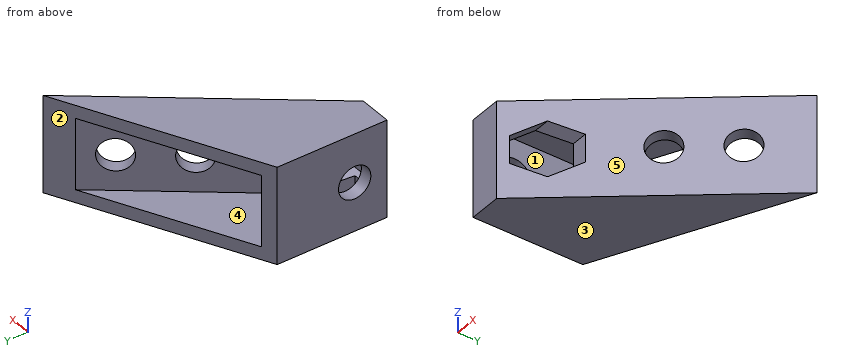
Autodesk Inventor part; units mm, degrees
ref_plane "YZ Plane" through (0, 0, 0) normal (1, 0, 0) x (0, 1, 0)
ref_plane "XZ Plane" through (0, 0, 0) normal (0, 1, 0) x (-1, 0, 0)
ref_plane "XY Plane" through (0, 0, 0) normal (0, 0, 1) x (1, 0, 0)
sketch "Skizze1" plane through (0, 0, 0) normal (0, 0, 1) x (1, 0, 0)
  line L0 (0, 0) -> (0, 17)
  line L1 (0, 0) -> (40, 0) construction
  line L2 (0, 0) -> (5, 0)
  line L3 (5, 0) -> (29.6265, 31.5204)
  line L4 (29.6265, 31.5204) -> (0, 17)
  dimension "d0" = 17
  dimension "d46" = 5
  dimension "d48" = 40
extrude "Extrusion1" add sketch "Skizze1" along normal blind 15
hole "Bohrung1" at (0, 5, 7.5) direction (1, 0, 0) diameter 5 end through all
shell "Wandstärke3" thickness 2 removed faces 2 at (9.8755, 21.8401, 5) at (3.6198, 7.5, 7.5084)
sketch "Skizze5" plane through (2, 2, 2) normal (1, 0, 0) x (0, 0, -1)
  circle A0 centre (-5.5, 3) radius 2.5
  line L0 (-3.35, -0.7239) -> (-7.65, -0.7239)
  line L1 (-7.65, -0.7239) -> (-9.8, 3)
  line L2 (-9.8, 3) -> (-7.65, 6.7239)
  line L3 (-7.65, 6.7239) -> (-3.35, 6.7239)
  line L4 (-3.35, 6.7239) -> (-1.2, 3)
  line L5 (-1.2, 3) -> (-3.35, -0.7239)
  point P0 (2, -2)
  dimension "d71" = 4.3
extrude "Extrusion4" cut sketch "Skizze5" along normal blind 10
hole "Bohrung6" at (22.4352, 25.5645, 7.5) direction (0.7880108, -0.6156615, 0) diameter 5 end through all
hole "Bohrung7" at (16.2786, 17.6844, 7.5) direction (0.7880108, -0.6156615, 0) diameter 5 end through all
properties part number "Befestigung"
The listing builds one solid part. Answer for the finished solid, in the listing's coordinates (mm). Face numbers are marked on the shaded views. A direction names the side the tool comes from. Coordinates: 2 decimals unless noted, no trailing zeros. Loops run counter-clockwise (first coordinate to the right, second up) from the corner with the lowest first, then second, coordinate; pieces in that order, holes last. Notation, with made-up numbers: (11.25, 50) - (37.25, 50) arc R12 cw to (37.25, 73) - close; hole circle Ø4 at (71.25, 30). An arc over 180 degrees is marked (long way). Use a Markdown table: item, result. Add a question column.
1) The part is cut by section B-B, the plane z = 8.5. Give the vertices of the cut face in (x, y), and give its area (3 significant figures).
2) Given pin 1 (3.5 mm diameter, centred on y = 8, z = 10, fed in from +X); pin 2 (4 mm diameter, centred on y = 5, z = 7.5, fed in from -X); pin 3 (8 mm diameter, centred on y = 15, z = 7.5, fed in from +X); pin 4 (1.3 mm diameter, centred on x = 10, z = 7, fed in from -Y), each flat-ended and moving along its own axis, determine where each tip first touches the part or whether it passes through.
3) Find the intervals of material crossed by line 1 (Z direction, x = 1.5, y = 5); line 2 (Z direction, x = 2.25, y = 15); line 3 (X direction, y = 13.5, z = 10.5), in increasing order.
4) The mould has two halves that part along X. Classify the marked faces 1, 2 and 3: released by +X, released by -X, zero draft, split by the parting line, or undercut.
5) For the marked faces 4 and 5, determine the directions among +Z, -Z, +X, -X, +Y, -Y from which every point of the face is accessible in a straight line to the end or side of a thin tool.
6) The part is cut by section C-C, the plane z = 12.5. Give the vertices of the cut face in (x, y), and give its area (3 significant figures).
7) The part is cut by section A-A, the plane x = 6.75. Give the vertices of the cut face in (y, z).
8) The part is cut by section D-D, the plane y = 7. Give the vertices of the cut face in (x, z).
Here are the results:
| question | item | result |
|---|---|---|
| 1 | outline | (0, 0) - (5, 0) - (6, 1.28) - (2, 1.28) - (2, 2.71) - (0, 2.71) - close; (0, 7.29) - (2, 7.29) - (2, 17.98) - (0, 17) - close; (9.28, 8.72) - (11.82, 8.72) - (16.44, 14.65) - (14.87, 15.88) - close; (17.69, 19.49) - (19.27, 18.26) - (22.6, 22.53) - (21.02, 23.76) - close; (23.85, 27.37) - (25.42, 26.14) - (29.63, 31.52) - (25.51, 29.5) - close |
| 1 | area | 67.2 mm^2 |
| 2 | pin 1 | stops at x = 12.62 |
| 2 | pin 2 | passes through |
| 2 | pin 3 | stops at x = 19.84 |
| 2 | pin 4 | stops at y = 8.72 |
| 3 | line 1 | z = 0 to 5, 10 to 15 |
| 3 | line 2 | z = 0 to 2, 13 to 15 |
| 3 | line 3 | x = 0 to 2, 13.01 to 15.55 |
| 4 | face 1 | undercut |
| 4 | face 2 | released by -X |
| 4 | face 3 | zero draft |
| 5 | face 4 | +Y |
| 5 | face 5 | +Z, -Z, +X, -Y |
| 6 | outline | (0, 0) - (5, 0) - (29.63, 31.52) - (25.51, 29.5) - (4.02, 2) - (2, 2) - (2, 17.98) - (0, 17) - close |
| 6 | area | 115 mm^2 |
| 7 | outline | (2.24, 0) - (20.31, 0) - (20.31, 2) - (5.49, 2) - (5.49, 3.48) - (5, 3.2) - (2.24, 4.79) - close; (2.24, 10.21) - (5, 11.8) - (5.49, 11.52) - (5.49, 13) - (20.31, 13) - (20.31, 15) - (2.24, 15) - close |
| 8 | outline | (0, 0) - (10.47, 0) - (10.47, 4.35) - (7.93, 4.35) - (7.93, 2) - (2, 2) - (2, 6) - (0, 6) - close; (0, 9) - (2, 9) - (2, 13) - (7.93, 13) - (7.93, 10.65) - (10.47, 10.65) - (10.47, 15) - (0, 15) - close |
